Source: CAD feature listing. Evaluate the final solid. Frame: model axes, mm. A direction names the side the tool comes from. Give positions to 0.01 mm unless a question says otherwise; leave off trailing zeros. Write each loop counter-clockwise with the first axis right and the second up, starting at its lowest first coordinate (ties: lowest second). Pieces come first, ordered by that corner, then holes. Notation, with made-up numbers: M 52,68 L 88,68 A26 ccw 88,102 Z; hole C -20,89 d11. An arc over 180 degrees is marked long. Return JSON: item names as keys, results as strings.
```python
from build123d import *

# Parameters (mm, degrees)
SKETCH1_W           = 31.8
SKETCH1_H           = 48
BOSS_EXTRUDE1_DEPTH = 15.8
SKETCH2_R           = 7.62
CUT_EXTRUDE1_DEPTH  = 12.7
SKETCH3_R           = 2.77815
SKETCH3_R_2         = 1.8415
CUT_EXTRUDE2_DEPTH  = 12.7
CUT_EXTRUDE3_DEPTH  = 1.905
SKETCH5_R           = 2.41
BOSS_EXTRUDE2_DEPTH = 1.905
SKETCH6_W           = 29.36
SKETCH6_H           = 13.36
SKETCH6_R           = 3.26
CUT_EXTRUDE4_DEPTH  = 1.905


with BuildPart() as part:
    # Sketch1 → Boss-Extrude1 (new body)
    with BuildSketch(Plane.XY):
        Rectangle(SKETCH1_W, SKETCH1_H)
    extrude(amount=BOSS_EXTRUDE1_DEPTH)

    # Sketch2 → Cut-Extrude1 (cut)
    with BuildSketch(Plane.XY.offset(15.8)):
        with Locations((0, 10.6)):
            Circle(SKETCH2_R)
        with BuildLine():
            Line((4.7625, -2.1), (4.7625, -14.8))
            ThreePointArc((4.7625, -14.8), (0, -19.5625), (-4.7625, -14.8))
            Line((-4.7625, -14.8), (-4.7625, -2.1))
            ThreePointArc((-4.7625, -2.1), (0, 2.6625), (4.7625, -2.1))
        make_face()
    extrude(amount=-CUT_EXTRUDE1_DEPTH, mode=Mode.SUBTRACT)

    # Sketch3 → Cut-Extrude2 (cut)
    with BuildSketch(Plane(origin=(0, 0, 0), x_dir=(-1, 0, 0), z_dir=(0, 0, -1))):
        with Locations((0, 10.6)):
            Circle(SKETCH3_R)
        with Locations((0, -2.1)):
            Circle(SKETCH3_R_2)
        with Locations((0, -14.8)):
            Circle(SKETCH3_R_2)
    extrude(amount=-CUT_EXTRUDE2_DEPTH, mode=Mode.SUBTRACT)

    # Sketch4 → Cut-Extrude3 (cut)
    with BuildSketch(Plane(origin=(0, 0, 0), x_dir=(-1, 0, 0), z_dir=(0, 0, -1))):
        with BuildLine():
            Line((4.7625, -14.8), (4.7625, -2.1))
            ThreePointArc((4.7625, -2.1), (0, 2.6625), (-4.7625, -2.1))
            Line((-4.7625, -2.1), (-4.7625, -14.8))
            ThreePointArc((-4.7625, -14.8), (0, -19.5625), (4.7625, -14.8))
        make_face()
    extrude(amount=-CUT_EXTRUDE3_DEPTH, mode=Mode.SUBTRACT)

    # Sketch5 → Boss-Extrude2 (add)
    with BuildSketch(Plane(origin=(0, 24, 0), x_dir=(1, 0, 0), z_dir=(0, 1, 0))):
        with Locations((-12, -3.9)):
            Circle(SKETCH5_R)
        with Locations((-12, -11.9)):
            Circle(SKETCH5_R)
        with Locations((-4, -3.9)):
            Circle(SKETCH5_R)
        with Locations((-4, -11.9)):
            Circle(SKETCH5_R)
        with Locations((4, -3.9)):
            Circle(SKETCH5_R)
        with Locations((4, -11.9)):
            Circle(SKETCH5_R)
        with Locations((12, -3.9)):
            Circle(SKETCH5_R)
        with Locations((12, -11.9)):
            Circle(SKETCH5_R)
    extrude(amount=BOSS_EXTRUDE2_DEPTH)

    # Sketch6 → Cut-Extrude4 (cut)
    with BuildSketch(Plane.XZ.offset(24)):
        with Locations((0, 7.9)):
            Rectangle(SKETCH6_W, SKETCH6_H)
        with Locations((-8, 7.9)):
            Circle(SKETCH6_R, mode=Mode.SUBTRACT)
        with Locations((0, 7.9)):
            Circle(SKETCH6_R, mode=Mode.SUBTRACT)
        with Locations((8, 7.9)):
            Circle(SKETCH6_R, mode=Mode.SUBTRACT)
    extrude(amount=-CUT_EXTRUDE4_DEPTH, mode=Mode.SUBTRACT)


solid = part.part
```
1) Cut plane B-B, the plane y = -11.5. Return the cut outline in (x, z) (1 decimal).
Numbers:
{"outline": "M -15.9,0 L -4.8,0 L -4.8,1.9 L 4.8,1.9 L 4.8,0 L 15.9,0 L 15.9,15.8 L 4.8,15.8 L 4.8,3.1 L -4.8,3.1 L -4.8,15.8 L -15.9,15.8 Z"}
2) Set-up query: faces 1 (the face through (0.1, -19.56, 9.54)), 2 (the face through (-4.762, -9, 1)), 3 (the face through (-1.7, 24.94, 3.18)). Return all of +Z, -Z, +X, -X, +Y, -Y with unobstructed straight access to the full face (end or side cutting, diameter ignored); none if empty.
Numbers:
{"face 1": "+Z", "face 2": "-Z", "face 3": "+Y"}
3) Draft query along X for faces 4 (the face through (8, -24, 8)), 5 (the face through (1.592, 24.939, 11.794)). Return one class per face: released by +X, released by -X, zero draft, split by the parting line, or undercut.
Numbers:
{"face 4": "zero draft", "face 5": "undercut"}
4) Cut plane C-C, the plane x = -12. Return the cut outline in (y, z) (3 decimals).
Numbers:
{"outline": "M -24,0 L 24,0 L 24,1.49 L 25.905,1.49 L 25.905,6.31 L 24,6.31 L 24,9.49 L 25.905,9.49 L 25.905,14.31 L 24,14.31 L 24,15.8 L -24,15.8 L -24,14.58 L -22.095,14.58 L -22.095,1.22 L -24,1.22 Z"}
5) Cut plane D-D, the plane z = 7.9. Return the cut outline in (x, y) (1 decimal).
Numbers:
{"outline": "M -15.9,-24 L -14.7,-24 L -14.7,-22.1 L -11.3,-22.1 L -11.3,-24 L -4.7,-24 L -4.7,-22.1 L -3.3,-22.1 L -3.3,-24 L 3.3,-24 L 3.3,-22.1 L 4.7,-22.1 L 4.7,-24 L 11.3,-24 L 11.3,-22.1 L 14.7,-22.1 L 14.7,-24 L 15.9,-24 L 15.9,24 L -15.9,24 Z; hole C 0,10.6 d15.2; hole M -4.8,-14.8 A4.8 ccw 4.8,-14.8 L 4.8,-2.1 A4.8 ccw -4.8,-2.1 Z"}
6) Cut plane A-A, the plane z = 3.9. Give the number of separate pieces and of enclosed holes in the cut face, then the cut area to 3 significant figures.
Numbers:
{"separate pieces": "1", "enclosed holes": "2", "area": "1,130 mm²"}
7) Line query: line 1 (Y direction, x = 0, z = 2.5) (1 decimal); line 2 (Y direction, x = 0, z = 11.25) (1 decimal); line 3 (Y direction, x = 0, z = 0.85). Output: solid intervals per line, ascending. Write a range as [from, to].
Numbers:
{"line 1": "y = [-22.1, -16.6], [-13, -3.9], [-0.3, 7.8], [13.4, 24]", "line 2": "y = [-22.1, -19.6], [2.7, 3], [18.2, 24]", "line 3": "y = [-24, -19.56], [2.66, 7.82], [13.38, 24]"}
8) Contact query for flat-ended pins moving along their axis: pin 1 Ø5 at (x, y) = (0, -2.1) entering from -Z (3 decimals); pin 2 Ø2 at (x, z) = (9, 9) entering from +Y; pin 3 Ø5 at (x, y) = (0, -8) entering from +Z. Output: stop coordinate, or through.
Numbers:
{"pin 1": "stops at z = 1.905", "pin 2": "stops at y = 24", "pin 3": "stops at z = 3.1"}
